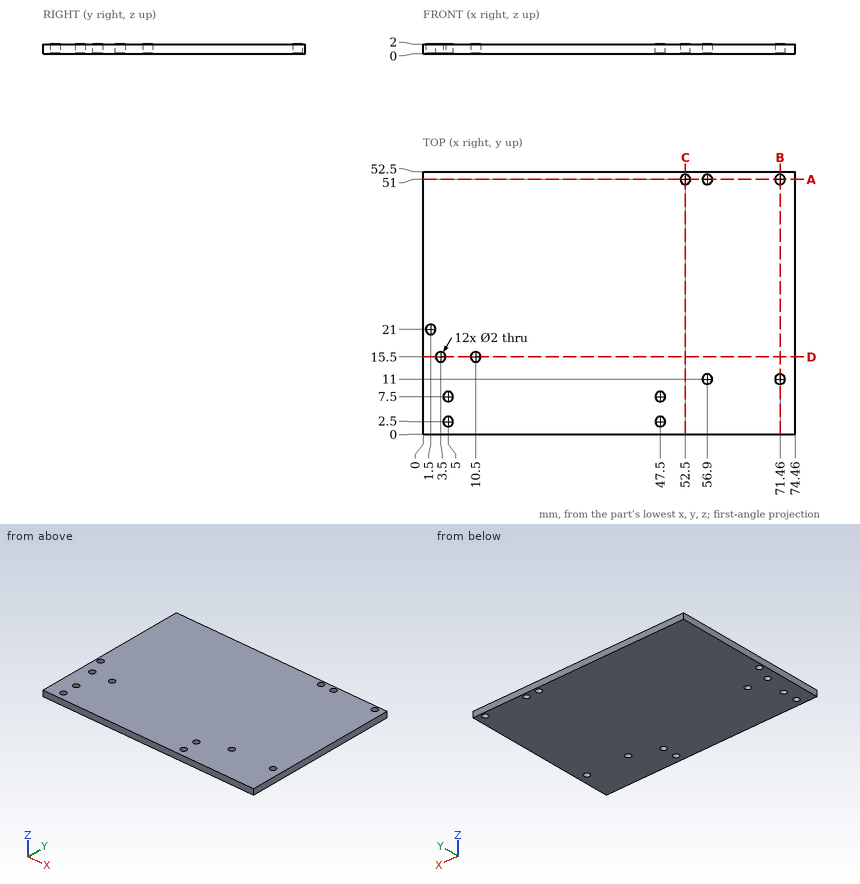
The drawing under review shows one solid part. Ordinate dimensions are in mm from its lowest x, y, z. Give positions to 0.01 mm unless a question says otherwise; leave off trailing zeros. Write each loop counter-clockwise with the first axis right and the second up, starting at its lowest first coordinate (ties: lowest second). Pieces come first, ordered by that corner, then holes.
1. Wall thickness on L1, parallel to Y at x = 56.9, z = 0.95; L2, parallel to Y at x = 5, z = 0.65; L3, parallel to X at y = 15.5, z = 1.05: over which ranges is each line inside the solid? List them lowest first.
2. For P1, Ø1.6, axis at x = 1.5, y = 21, coming from the +Z side, flat-tipped, find the tip position at first contact; note if it passes through.
3. Add section D-D, the plane y = 15.5. Write out the cut boundary in (x, z).
4. Add section C-C, the plane x = 52.5. Write out the cut boundary in (y, z), plus the area to 3 significant figures.
5. Add section B-B, the plane x = 71.46. Write out the cut boundary in (y, z).
6. Add section A-A, the plane y = 51. Write out the cut boundary in (x, z), plus the area to 3 significant figures.
Worked answers:
1. L1: y = 0 to 10, 12 to 50, 52 to 52.5
1. L2: y = 0 to 1.5, 3.5 to 6.5, 8.5 to 52.5
1. L3: x = 0 to 2.5, 4.5 to 9.5, 11.5 to 74.46
2. P1: passes through
3. outline: (0, 0) - (2.5, 0) - (2.5, 2) - (0, 2) - close; (4.5, 0) - (9.5, 0) - (9.5, 2) - (4.5, 2) - close; (11.5, 0) - (74.46, 0) - (74.46, 2) - (11.5, 2) - close
4. outline: (0, 0) - (50, 0) - (50, 2) - (0, 2) - close; (52, 0) - (52.5, 0) - (52.5, 2) - (52, 2) - close
4. area: 101 mm2
5. outline: (0, 0) - (10, 0) - (10, 2) - (0, 2) - close; (12, 0) - (50, 0) - (50, 2) - (12, 2) - close; (52, 0) - (52.5, 0) - (52.5, 2) - (52, 2) - close
6. outline: (0, 0) - (51.5, 0) - (51.5, 2) - (0, 2) - close; (53.5, 0) - (55.9, 0) - (55.9, 2) - (53.5, 2) - close; (57.9, 0) - (70.46, 0) - (70.46, 2) - (57.9, 2) - close; (72.46, 0) - (74.46, 0) - (74.46, 2) - (72.46, 2) - close
6. area: 137 mm2
